```python
from build123d import *

# Parameters (mm, degrees)
SKETCH3_W           = 11.5
SKETCH3_H           = 11.5
BOSS_EXTRUDE1_DEPTH = 12.5
SKETCH4_R           = 1.55
CUT_EXTRUDE1_DEPTH  = 3
CUT_EXTRUDE2_DEPTH  = 11.5
SKETCH6_W           = 5.3
SKETCH6_H           = 10.5
CUT_EXTRUDE3_DEPTH  = 6.75


with BuildPart() as part:
    # Sketch3 → Boss-Extrude1 (new body)
    with BuildSketch(Plane(origin=(0, 0, 0), x_dir=(1, 0, 0), z_dir=(0, 1, 0))):
        Rectangle(SKETCH3_W, SKETCH3_H)
    extrude(amount=BOSS_EXTRUDE1_DEPTH)

    # Sketch4 → Cut-Extrude1 (cut, through all)
    with BuildSketch(Plane(origin=(0, 10.5, 0), x_dir=(1, 0, 0), z_dir=(0, 1, 0))):
        Circle(SKETCH4_R)
    extrude(amount=CUT_EXTRUDE1_DEPTH, mode=Mode.SUBTRACT)

    # Sketch5 → Cut-Extrude2 (cut, through all)
    with BuildSketch(Plane(origin=(0, 10.5, 0), x_dir=(1, 0, 0), z_dir=(0, 1, 0))):
        Polygon((3.059956427, 0), (1.529978213, 2.65), (-1.529978213, 2.65), (-3.059956427, 0), (-1.529978213, -2.65), (1.529978213, -2.65), align=None)
    extrude(amount=-CUT_EXTRUDE2_DEPTH, mode=Mode.SUBTRACT)

    # Sketch6 → Cut-Extrude3 (cut, through all)
    with BuildSketch(Plane(origin=(0, 0, 0), x_dir=(0, 0, -1), z_dir=(1, 0, 0))):
        with Locations((0, 5.25)):
            Rectangle(SKETCH6_W, SKETCH6_H)
    extrude(amount=-CUT_EXTRUDE3_DEPTH, mode=Mode.SUBTRACT)


solid = part.part
```
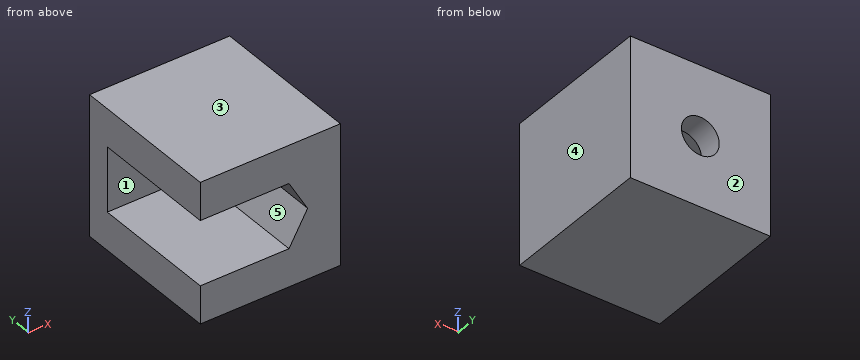
Here's how the part is built. I have some questions about the finished solid (model axes, mm). Face numbers are marked on the shaded views. A direction names the side the tool comes from. Round coordinates to 2 decimals unless told otherwise and drop trailing zeros. Loops run counter-clockwise (first coordinate to the right, second up) from the corner with the lowest first, then second, coordinate; pieces in that order, holes last.
1. Will these pins go through, and if not, where does the flat tip stop? pin 1 (3 mm diameter, centred on x = 0, z = 0, fed in from +Y); pin 2 (1 mm diameter, centred on y = 8, z = -2, fed in from -X); pin 3 (4 mm diameter, centred on x = -0.5, z = -0.5, fed in from -Y).
Answers:
pin 1: passes through
pin 2: stops at x = 1.62
pin 3: stops at y = 10.5
2. Suppose I cut it at D-D, the plane x = 2.5. Please give me the cut outline in (y, z), and give its area (3 significant figures).
Answers:
outline: (0, -5.75) - (12.5, -5.75) - (12.5, 5.75) - (0, 5.75) - (0, 0.97) - (10.5, 0.97) - (10.5, -0.97) - (0, -0.97) - close
area: 123 mm2
3. Suppose I cut it at A-A, the plane x = 0. Please give me the cut outline in (y, z), and give its area (3 significant figures).
Answers:
outline: (0, -5.75) - (12.5, -5.75) - (12.5, -1.55) - (10.5, -1.55) - (10.5, -2.65) - (0, -2.65) - close; (0, 2.65) - (10.5, 2.65) - (10.5, 1.55) - (12.5, 1.55) - (12.5, 5.75) - (0, 5.75) - close
area: 81.9 mm2
4. For the marked faces 4 and 5, which set-ups out of +Z, -Z, +X, -X, +Y, -Y let a thin tool reach every point of the face, with its end or its side?
Answers:
face 4: +Z, -Z, +X, +Y, -Y
face 5: -X, -Y
5. Thinking about a two-plate mould opening in Z: for the marked faces 1, 2 and 3, which applies, released by +Z, released by -Z, zero draft, split by the parting line, or undercut?
Answers:
face 1: undercut
face 2: zero draft
face 3: released by +Z
6. Suppose I cut it at B-B, the plane y = 8.75. Please give me the cut outline in (x, z).
Answers:
outline: (-5.75, -5.75) - (5.75, -5.75) - (5.75, 5.75) - (-5.75, 5.75) - (-5.75, 2.65) - (1.53, 2.65) - (3.06, 0) - (1.53, -2.65) - (-5.75, -2.65) - close
7. Suppose I cut it at C-C, the plane z = -1. Please give me the cut outline in (x, y), and give its area (3 significant figures).
Answers:
outline: (-5.75, 10.5) - (-1.18, 10.5) - (-1.18, 12.5) - (-5.75, 12.5) - close; (1.18, 10.5) - (2.48, 10.5) - (2.48, 0) - (5.75, 0) - (5.75, 12.5) - (1.18, 12.5) - close
area: 52.6 mm2
8. If I drill on probe 1 along X at (y, z) = (11.7, 0); probe 2 along Z at (x, y) = (0.75, 3.5), over which ranges is the centre line in solid material (lowest first)?
Answers:
probe 1: x = -5.75 to -1.55, 1.55 to 5.75
probe 2: z = -5.75 to -2.65, 2.65 to 5.75
